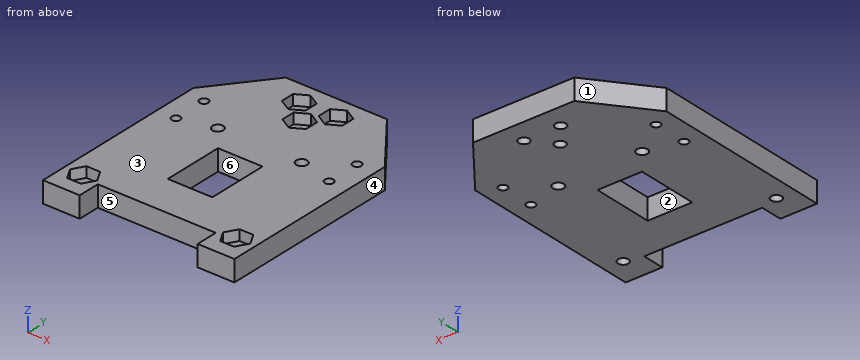
```python
from build123d import *

# Parameters (mm, degrees)
ESBO_O1_R                = 2
ESBO_O1_R_2              = 2.086716092
ESBO_O1_R_3              = 2.086717953
RESSALTO_EXTRUS_O1_DEPTH = 8
ESBO_O4_R                = 1.65
CORTE_EXTRUS_O1_DEPTH    = 100.298791533
CORTE_EXTRUS_O2_DEPTH    = 4


with BuildPart() as part:
    # Esboço1 → Ressalto-extrusão1 (new body)
    with BuildSketch(Plane.XY):
        Polygon((19.311716217, 92), (-19.311716217, 92), (-36.5, 70), (-36.5, 0), (-22.499999998, 0), (-22.499999998, 8.400000004), (22.499999998, 8.400000004), (22.499999998, 0), (36.5, 0), (36.5, 70), align=None)
        with Locations((0, 75)):
            Circle(ESBO_O1_R, mode=Mode.SUBTRACT)
        with Locations((-7, 83.3)):
            Circle(ESBO_O1_R, mode=Mode.SUBTRACT)
        with Locations((7, 83.3)):
            Circle(ESBO_O1_R, mode=Mode.SUBTRACT)
        with Locations((-29.2, 10)):
            Circle(ESBO_O1_R, mode=Mode.SUBTRACT)
        with Locations((29.2, 10)):
            Circle(ESBO_O1_R, mode=Mode.SUBTRACT)
        with Locations((-16, 56.354540575)):
            Circle(ESBO_O1_R_2, mode=Mode.SUBTRACT)
        with Locations((16, 56.354540575)):
            Circle(ESBO_O1_R_3, mode=Mode.SUBTRACT)
        Polygon((0, 47.257129716), (8.5, 47.257129716), (8.5, 23.917682695), (0, 23.917682695), (-8.5, 23.917682695), (-8.5, 47.257129716), align=None, mode=Mode.SUBTRACT)
    extrude(amount=RESSALTO_EXTRUS_O1_DEPTH)

    # Esboço4 → Corte-extrusão1 (cut, through all)
    with BuildSketch(Plane.XY.offset(8)):
        with Locations((-29.2, 66)):
            Circle(ESBO_O4_R)
        with Locations((-29.2, 53)):
            Circle(ESBO_O4_R)
        with Locations((29.2, 53)):
            Circle(ESBO_O4_R)
        with Locations((29.2, 66)):
            Circle(ESBO_O4_R)
    extrude(amount=-CORTE_EXTRUS_O1_DEPTH, mode=Mode.SUBTRACT)

    # Esboço5 → Corte-extrusão2 (cut)
    with BuildSketch(Plane.XY.offset(8)):
        Polygon((4.5, 72.401923789), (4.5, 77.598076211), (0, 80.196152423), (-4.5, 77.598076211), (-4.5, 72.401923789), (0, 69.803847577), align=None)
        Polygon((-26.601923789, 14.5), (-31.798076211, 14.5), (-34.396152423, 10), (-31.798076211, 5.5), (-26.601923789, 5.5), (-24.003847577, 10), align=None)
        Polygon((-11.5, 80.701923789), (-7, 78.103847577), (-2.5, 80.701923789), (-2.5, 85.898076211), (-7, 88.496152423), (-11.5, 85.898076211), align=None)
        Polygon((11.5, 80.701923789), (11.5, 85.898076211), (7, 88.496152423), (2.5, 85.898076211), (2.5, 80.701923789), (7, 78.103847577), align=None)
        Polygon((31.798076211, 5.5), (34.396152423, 10), (31.798076211, 14.5), (26.601923789, 14.5), (24.003847577, 10), (26.601923789, 5.5), align=None)
    extrude(amount=-CORTE_EXTRUS_O2_DEPTH, mode=Mode.SUBTRACT)


solid = part.part
```
CAD build for the part. Positions are in the model's coordinates, mm. Face numbers are marked on the shaded views. A direction names the side the tool comes from. Round coordinates to 2 decimals unless told otherwise and drop trailing zeros. Order: outer loops, then holes, each group sorted by start corner. A loop starts at its lowest first (then second) coordinate and runs counter-clockwise, first axis right, second up.
Item 1: Saw through at A-A on y = 53. Write the cut outline in (x, z), then the cut area to 3 significant figures.
Item 2: Saw through at C-C on z = 2. State how many separate pieces and enclosed holes the cut face has, then the cut area to 3 significant figures.
Item 3: Pin check, flat tips, straight feed: pin 1 (2 mm diameter, centred on x = -3.5, y = 72.5, fed in from -Z); pin 2 (1.5 mm diameter, centred on x = -10.5, z = 3, fed in from -Y); pin 3 (3 mm diameter, centred on y = 84, z = 5.5, fed in from -X); pin 4 (2.5 mm diameter, centred on x = 28, y = 8.5, fed in from +Z). Stop position of each tip, or through.
Item 4: Saw through at B-B on x = 29.2. Write the cut outline in (y, z), then the cut area to 3 significant figures.
Item 5: Probe line 1 along Y through (x, z) = (-16, 4.75); line 2 along X through (y, z) = (51.5, 7.5); line 3 along Y through (x, z) = (5.5, 3). List the from-to ranges inside material, lowest first.
Item 6: Saw through at D-D on y = 83.3. Write the cut outline in (x, z), then the cut area to 3 significant figures.
Item 7: Tool access for the marked faces 4, 5 and 6: list every direction of +Z, -Z, +X, -X, +Y, -Y with a clear straight run to the whole face (end or side of a thin tool).
Item 8: Mould opens along X. For the marked faces 1, 2 and 3 say: pulls with the +X half, pulls with the -X half, needs draft (parallel to the pull), parting line crosses it, or undercut.
Reported:
1. outline: (-36.5, 0) - (-30.85, 0) - (-30.85, 8) - (-36.5, 8) - close; (-27.55, 0) - (27.55, 0) - (27.55, 8) - (-27.55, 8) - close; (30.85, 0) - (36.5, 0) - (36.5, 8) - (30.85, 8) - close
1. area: 531 mm2
2. separate pieces: 1
2. enclosed holes: 12
2. area: 5,440 mm2
3. pin 1: stops at z = 0
3. pin 2: stops at y = 8.4
3. pin 3: stops at x = -26.73
3. pin 4: stops at z = 4
4. outline: (0, 0) - (8, 0) - (8, 4) - (5.5, 4) - (5.5, 8) - (0, 8) - close; (12, 0) - (51.35, 0) - (51.35, 8) - (14.5, 8) - (14.5, 4) - (12, 4) - close; (54.65, 0) - (64.35, 0) - (64.35, 8) - (54.65, 8) - close; (67.65, 0) - (79.34, 0) - (79.34, 8) - (67.65, 8) - close
4. area: 530 mm2
5. line 1: y = 8.4 to 54.27, 58.44 to 92
5. line 2: x = -36.5 to -29.89, -28.51 to 28.51, 29.89 to 36.5
5. line 3: y = 8.4 to 23.92, 47.26 to 81.98, 84.62 to 92
6. outline: (-26.11, 0) - (-9, 0) - (-9, 4) - (-11.5, 4) - (-11.5, 8) - (-26.11, 8) - close; (-5, 0) - (5, 0) - (5, 4) - (2.5, 4) - (2.5, 8) - (-2.5, 8) - (-2.5, 4) - (-5, 4) - close; (9, 0) - (26.11, 0) - (26.11, 8) - (11.5, 8) - (11.5, 4) - (9, 4) - close
6. area: 314 mm2
7. face 4: +Z, -Z, +X, +Y, -Y
7. face 5: +Z, -Z, -Y
7. face 6: +Z, -Z
8. face 1: pulls with the -X half
8. face 2: undercut
8. face 3: needs draft
